Part print with two shaded views. Sizes in mm from the minimum x, y, z corner. A direction names the side the tool comes from. Coordinates: 2 decimals unless noted, no trailing zeros. Loops run counter-clockwise (first coordinate to the right, second up) from the corner with the lowest first, then second, coordinate; pieces in that order, holes last. Notation, with made-up numbers: (79, 40) -> (103, 40) arc R10 cw to (103, 58) -> close; hole circle Ø11 at (82.25, 21). An arc over 180 degrees is marked (long way). Write each question's results on one line, items separated by ' | '.
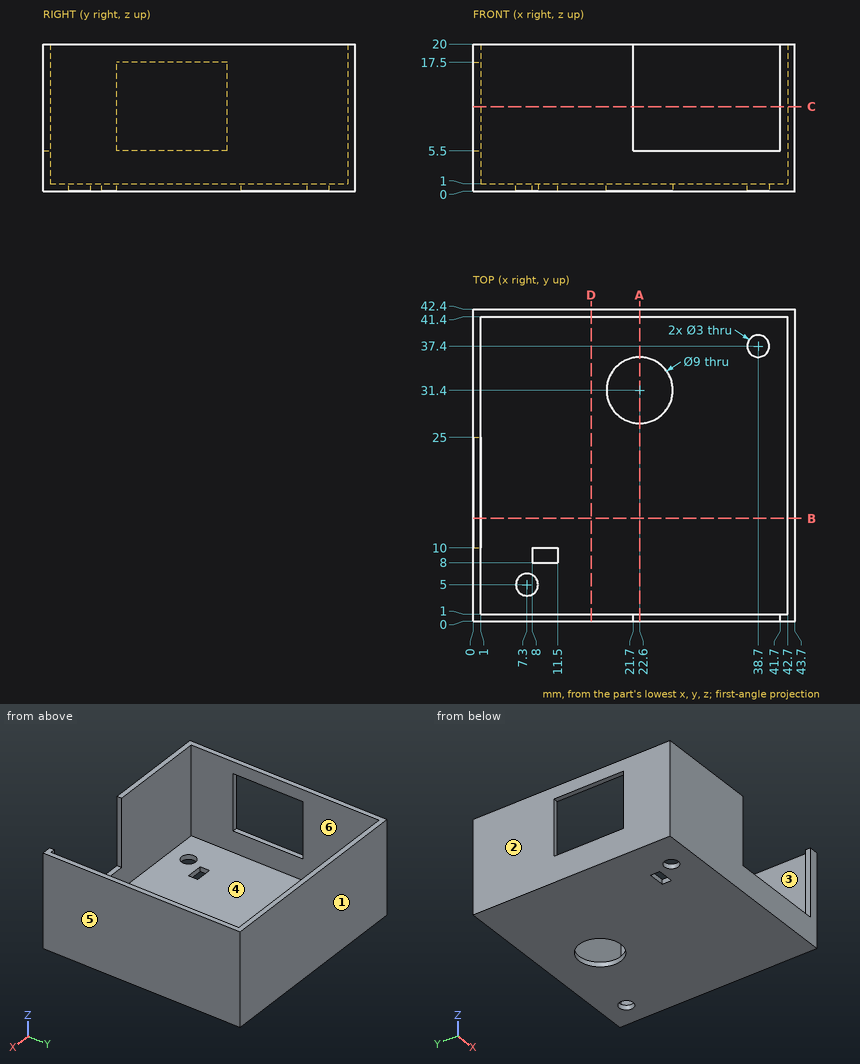
Q1. Cut at A-A on x = 22.6. Write the cut outline in (y, z).
Results are:
outline: (0, 0) -> (26.9, 0) -> (26.9, 1) -> (1, 1) -> (1, 5.5) -> (0, 5.5) -> close; (35.9, 0) -> (42.4, 0) -> (42.4, 20) -> (41.4, 20) -> (41.4, 1) -> (35.9, 1) -> close
Q2. Which spindle directions (+Z, -Z, +X, -X, +Y, -Y) get a long thin tool onto all of the face, cutting with end or side? Do the marked faces 5 and 6. Say none if no direction does.
Results are:
face 5: +Z, -Z, +X, +Y, -Y | face 6: +Z
Q3. Cut at B-B on y = 14. Write the cut outline in (x, z).
Results are:
outline: (0, 0) -> (43.7, 0) -> (43.7, 20) -> (42.7, 20) -> (42.7, 1) -> (1, 1) -> (1, 5.5) -> (0, 5.5) -> close; (0, 17.5) -> (1, 17.5) -> (1, 20) -> (0, 20) -> close
Q4. Cut at D-D on x = 16. Write the cut outline in (y, z).
Results are:
outline: (0, 0) -> (42.4, 0) -> (42.4, 20) -> (41.4, 20) -> (41.4, 1) -> (1, 1) -> (1, 20) -> (0, 20) -> close
Q5. Pull direction X, two halves, no side cores. Call the marked faces 1, 2, 3 and 4: +X half, -X half, draft (parallel to the pull), parting line (faces both ways), or undercut.
Results are:
face 1: draft | face 2: -X half | face 3: undercut | face 4: undercut
Q6. Wall check: L1, parallel to Y at x = 22.6, z = 0.6; L2, parallel to Y at x = 7.3, z = 0.75; L3, parallel to X at y = 24, z = 1.5. Give the ranges that are in metal, low to high. Write a range as from..to.
Results are:
L1: 0..26.9, 35.9..42.4 | L2: 0..3.5, 6.5..42.4 | L3: 0..1, 42.7..43.7
Q7. Cut at C-C on z = 11.5. Write the cut outline in (x, y).
Results are:
outline: (0, 0) -> (21.7, 0) -> (21.7, 1) -> (1, 1) -> (1, 10) -> (0, 10) -> close; (0, 25) -> (1, 25) -> (1, 41.4) -> (42.7, 41.4) -> (42.7, 1) -> (41.7, 1) -> (41.7, 0) -> (43.7, 0) -> (43.7, 42.4) -> (0, 42.4) -> close
Q8. Drop flat-ended pins along their axis: pin 1 (3 mm diameter, centred on x = 34.5, z = 8, fed in from -Y); pin 2 (0.8 mm diameter, centred on x = 29, y = 0.5, fed in from +Z). Give the stop position or say it passes through.
Results are:
pin 1: y = 41.4 | pin 2: z = 5.5
